from build123d import *

# Parameters (mm, degrees)
SKETCH1_R               = 8
BOSS_EXTRUDE1_DEPTH     = 30
BOSS_EXTRUDE1_2_DEPTH   = 30
SKETCH2_W               = 30
SKETCH2_H               = 30
CUT_EXTRUDE1_DEPTH      = 30
CHAMFER1_SIZE           = 3
FILLET1_R               = 3
FILLET2_R               = 3
CUT_EXTRUDE2_DEPTH      = 30
CUT_EXTRUDE2_DEPTH_BACK = 30
SKETCH3_R               = 1.75
CUT_EXTRUDE3_DEPTH      = 50
CUT_EXTRUDE3_DEPTH_BACK = 30
SKETCH4_R               = 3
CUT_EXTRUDE4_DEPTH      = 88.933914818
CUT_EXTRUDE4_DEPTH_BACK = 88.933914818
SKETCH5_R               = 1.75
BOSS_EXTRUDE2_DEPTH     = 5
FILLET3_R               = 3
FILLET4_R               = 3
FILLET5_R               = 3
CHAMFER5_SIZE           = 5


with BuildPart() as part:
    # Sketch1 → Boss-Extrude1 (new body)
    with BuildSketch(Plane(origin=(0, 0, 0), x_dir=(1, 0, 0), z_dir=(0, 1, 0))):
        with Locations(Location((0.707106781, 0, 0), (0, 0, 270))):
            Circle(SKETCH1_R)
    extrude(amount=BOSS_EXTRUDE1_DEPTH)



with BuildPart() as body_2:
    # Sketch1 → Boss-Extrude1 2 (new body)
    with BuildSketch(Plane(origin=(0, 0, 0), x_dir=(1, 0, 0), z_dir=(0, 1, 0))):
        Polygon((-65, 21.062445841), (-65, -21.062445841), (-21.005807434, -21.062445841), (-21.005807434, -30), (-15, -30), (-15, -21.062445841), (-36.062445841, 0), (-15, 21.062445841), (-15, 30), (-22, 30), (-22, 21.062445841), align=None)
    extrude(amount=BOSS_EXTRUDE1_2_DEPTH)

    # Sketch2 → Cut-Extrude1 (cut)
    with BuildSketch(Plane(origin=(0, 30, 0), x_dir=(1, 0, 0), z_dir=(0, 1, 0))):
        with Locations((-56.062445841, 0)):
            Rectangle(SKETCH2_W, SKETCH2_H)
    extrude(amount=-CUT_EXTRUDE1_DEPTH, mode=Mode.SUBTRACT)

    # Chamfer1
    chamfer1_edges = [body_2.edges().sort_by_distance(p)[0] for p in [
        (-21.005807434, 15, 21.062445841),
        (-22, 15, -21.062445841),
    ]]
    chamfer(chamfer1_edges, length=CHAMFER1_SIZE)

    # Fillet1
    fillet1_edges = [body_2.edges().sort_by_distance(p)[0] for p in [
        (-36.062445841, 15, 0),
        (-15, 15, 21.062445841),
        (-15, 15, -21.062445841),
        (-41.062445841, 15, 15),
        (-41.062445841, 15, -15),
    ]]
    fillet(fillet1_edges, radius=FILLET1_R)

    # Fillet2
    fillet2_edges = [body_2.edges().sort_by_distance(p)[0] for p in [
        (-15, 15, 30),
        (-21.005807434, 15, 30),
        (-65, 15, 21.062445841),
        (-65, 15, -21.062445841),
        (-22, 15, -30),
        (-15, 15, -30),
        (-65, 15, 15),
        (-65, 15, -15),
    ]]
    fillet(fillet2_edges, radius=FILLET2_R)

    # Sketch3 → Cut-Extrude2 (cut, two sides: drawn at the far end of the back side and taken through both)
    with BuildSketch(Plane.ZY.offset(22).offset(-CUT_EXTRUDE2_DEPTH_BACK)):
        with Locations(Location((-25, 15, 0), (0, 0, 57.605534529))):
            Circle(SKETCH3_R)
        with Locations(Location((25, 15, 0), (0, 0, 122.394465471))):
            Circle(SKETCH3_R)
    extrude(amount=CUT_EXTRUDE2_DEPTH + CUT_EXTRUDE2_DEPTH_BACK, mode=Mode.SUBTRACT)

    # Sketch4 → Cut-Extrude3 (cut, two sides: drawn at the far end of the back side and taken through both)
    with BuildSketch(Plane.XY.offset(-15).offset(-CUT_EXTRUDE3_DEPTH_BACK)):
        with Locations(Location((-55.062445841, 15.983841749, 0), (0, 0, 180))):
            Circle(SKETCH4_R)
    extrude(amount=CUT_EXTRUDE3_DEPTH + CUT_EXTRUDE3_DEPTH_BACK, mode=Mode.SUBTRACT)

    # Sketch5 → Cut-Extrude4 (cut, two sides: drawn at the far end of the back side and taken through both)
    with BuildSketch(Plane(origin=(0, 0, -21.062445841), x_dir=(-1, 0, 0), z_dir=(0, 0, -1)).offset(-CUT_EXTRUDE4_DEPTH_BACK)):
        with Locations((41, 15)):
            Circle(SKETCH5_R)
    extrude(amount=CUT_EXTRUDE4_DEPTH + CUT_EXTRUDE4_DEPTH_BACK, mode=Mode.SUBTRACT)


with BuildPart() as part_1:
    add(part.part)

    add(body_2.part)  # Boss-Extrude2 merges body 2
    # Sketch6 → Boss-Extrude2 (add)
    with BuildSketch(Plane(origin=(0, 0, 0), x_dir=(1, 0, 0), z_dir=(0, 1, 0))):
        Polygon((-15, 15), (15, 15), (15, -15), (-15, -15), (-15, -24.652543264), (-37.297750688, -1.415722551), (-37.297750688, 2.803501212), (-15, 23.928760824), align=None)
    extrude(amount=BOSS_EXTRUDE2_DEPTH)

    # Fillet3
    fillet3_edges = [part_1.edges().sort_by_distance(p)[0] for p in [
        (0.707106781, 30, -8),
    ]]
    fillet(fillet3_edges, radius=FILLET3_R)

    # Fillet4
    fillet4_edges = [part_1.edges().sort_by_distance(p)[0] for p in [
        (15, 2.5, 15),
        (15, 2.5, -15),
    ]]
    fillet(fillet4_edges, radius=FILLET4_R)

    # Fillet5
    fillet5_edges = [part_1.edges().sort_by_distance(p)[0] for p in [
        (0.707106781, 5, -8),
    ]]
    fillet(fillet5_edges, radius=FILLET5_R)

    # Chamfer5
    chamfer5_edges = [part_1.edges().sort_by_distance(p)[0] for p in [
        (-15, 2.5, -15),
        (-15, 2.5, 15),
    ]]
    chamfer(chamfer5_edges, length=CHAMFER5_SIZE)


solid = part_1.part
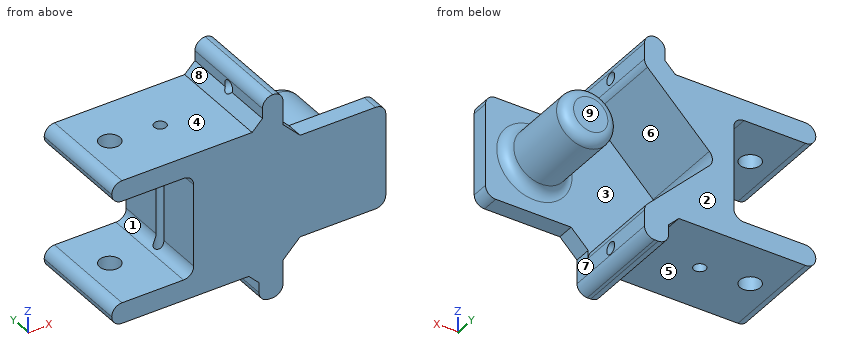
Read the model definition and answer for the solid it produces. Units are mm, in the model's axes. Face numbers are marked on the shaded views. A direction names the side the tool comes from. Give positions to 0.01 mm unless a question says otherwise; leave off trailing zeros. Write each loop counter-clockwise with the first axis right and the second up, starting at its lowest first coordinate (ties: lowest second). Pieces come first, ordered by that corner, then holes. Notation, with made-up numbers: (37.5, -32) -> (49.5, -32) arc R16 ccw to (49.5, -25) -> close; hole circle Ø3 at (-18, 34). An arc over 180 degrees is marked (long way). Answer as a JSON object with one key per item and string values. Group by question number.
1) The mould has two halves that part along X. Classify the marked faces 6, 7, 8 and 9: +X half, -X half, draft (parallel to the pull), parting line (faces both ways), or undercut.
2) A tool of negligible diameter and unlimited length cuts with its end or side. For the marked faces 1, 2, 3, 4 and 5, from which of +Z, -Z, +X, -X, +Y, -Y can it reach the whole face along a straight path? Write none if from no direction.
3) Find section B-B (x = -49). Write down the section's boundary in (y, z), and give its area (3 significant figures).
4) Find section D-D (z = 0). Write down the section's boundary in (x, y).
5) Each of these flat-tipped pins is pushed along its axis until it touches: P1, Ø1.5, axis at x = -4, y = 3, coming from the -Z side; P2, Ø4, axis at y = 15.5, z = -4, coming from the -X side; P3, Ø14.5, axis at x = -55.5, y = 10, coming from the +Z side; P4, Ø10, axis at x = -16.5, y = 13.5, coming from the -Z side. Where does it stop, or does it pass through?
6) Consider L1, parallel to Z at x = -20, y = 15; L2, parallel to Z at x = -52.5, y = 21.5; L3, parallel to Y at x = -41, z = -5.5. Determine where each line is inside the solid, lowest interval first. Write a range as from..to.
7) Find section A-A (z = 25). Write down the section's boundary in (x, y), and give its area (3 significant figures).
Values follow:
{
 "1": {"face 6": "undercut", "face 7": "+X half", "face 8": "-X half", "face 9": "draft"},
 "2": {"face 1": "-X, +Y, -Y", "face 2": "+Z, -Z, +X, -X, +Y", "face 3": "+Y", "face 4": "+Z, -X, +Y, -Y", "face 5": "-Z, -X, +Y, -Y"},
 "3": {"outline": "(0, -21.06) -> (30, -21.06) -> (30, -15) -> (0, -15) -> close; (0, 15) -> (30, 15) -> (30, 21.06) -> (0, 21.06) -> close", "area": "364 mm2"},
 "4": {"outline": "(-41.06, 0) -> (15, 0) -> (15, 5) -> (11.71, 5) arc R3 cw to (8.71, 8) -> (8.71, 27) arc R3 ccw to (5.71, 30) -> (-4.29, 30) arc R3 ccw to (-7.29, 27) -> (-7.29, 8) arc R3 cw to (-10.29, 5) -> (-34.82, 5) -> (-34.82, 30) -> (-41.06, 30) -> (-41.06, 16.75) arc R1.75 cw (long way) to (-41.06, 13.25) -> close"},
 "5": {"P1": "stops at z = -15", "P2": "stops at x = -41.06", "P3": "stops at z = 21.06", "P4": "stops at z = -30"},
 "6": {"L1": "z = -29.83..-26.75, -23.25..-16.06, 16.06..23.25, 26.75..29.24", "L2": "z = -21.06..-15, 15..21.06", "L3": "y = 0..13.25, 16.75..30"},
 "7": {"outline": "(-21.01, 0) -> (-15, 0) -> (-15, 13.25) -> (-21.01, 13.25) -> close; (-21.01, 16.75) -> (-15, 16.75) -> (-15, 30) -> (-21.01, 30) -> close", "area": "159 mm2"}
}
